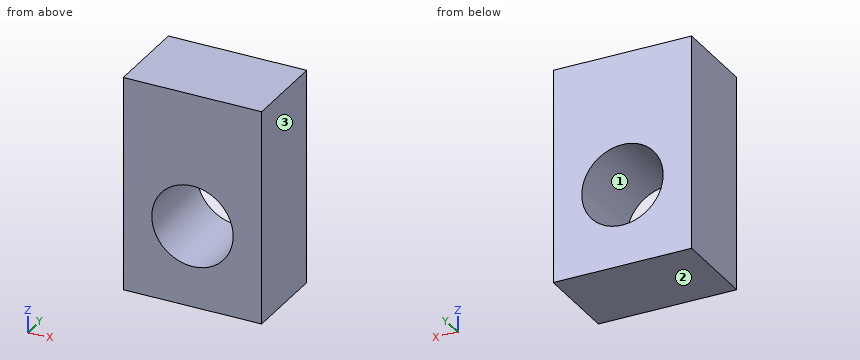
Autodesk Fusion 360 part; units mm, degrees
sketch "Sketch1" plane through (0, 0, 0) normal (0, 1, 0) x (1, 0, 0)
  line L0 (0, 0) -> (5.1, 0)
  line L1 (5.1, 0) -> (5.1, -7.9)
  line L2 (5.1, -7.9) -> (0, -7.9)
  line L3 (0, -7.9) -> (0, 0)
  point P0 (2.55, -3)
  dimension "d1" = 5.1
  dimension "d2" = 7.9
  dimension "d5" = 2.55
  dimension "d6" = 3
extrude "Extrude1" add sketch "Sketch1" along normal blind 3.2
hole "Hole1" at (2.55, 0, 3) direction (0, 1, 0) diameter 3 depth 8 tip angle 118
equation "d5 = ( 5.1 / 2 ) * 1 mm"
The model under review builds one solid part; all positions refer to its coordinate system, in mm. Face numbers are marked on the shaded views. Give positions to 0.01 mm unless a question says otherwise; leave off trailing zeros. Loops run counter-clockwise (first coordinate to the right, second up) from the corner with the lowest first, then second, coordinate; pieces in that order, holes last. Notation, with made-up numbers: (50.25, -18.5) -> (72.25, -18.5) arc R14 ccw to (72.25, -8.5) -> close; hole circle Ø2 at (37.5, 22.25). An arc over 180 degrees is marked (long way). Put each result on its own line as item: value. Start each with the question number.
1. We need section C-C on y = 0.35. State the section outline as (x, z) points.
2. Mouldability with a two-part tool opening along X and no side actions: class the marked faces 1, 2 and 3 as released by +X, released by -X, zero draft, split by the parting line, or undercut.
3. We need section A-A on z = 3. State the section outline as (x, y) points.
4. Clearance check with a flat-ended pin moving along its axis: P1, Ø2.5, axis at x = 2.55, z = 3, coming from the +Y side. State where the tip first meets the part, or that it passes through.
5. We need section B-B on x = 2.55. State the section outline as (y, z) points.
6. Wall thickness on probe 1 along X at (y, z) = (1.8, 3); probe 2 along Z at (x, y) = (2.55, 1.9); probe 3 along Z at (x, y) = (3, 0.75): over which ranges is each line inside the solid? List them lowest first.
Determined:
1. outline: (0, 0) -> (5.1, 0) -> (5.1, 7.9) -> (0, 7.9) -> close; hole circle Ø3 at (2.55, 3)
2. face 1: undercut
2. face 2: zero draft
2. face 3: released by +X
3. outline: (0, 0) -> (1.05, 0) -> (1.05, 3.2) -> (0, 3.2) -> close; (4.05, 0) -> (5.1, 0) -> (5.1, 3.2) -> (4.05, 3.2) -> close
4. P1: through
5. outline: (0, 0) -> (3.2, 0) -> (3.2, 1.5) -> (0, 1.5) -> close; (0, 4.5) -> (3.2, 4.5) -> (3.2, 7.9) -> (0, 7.9) -> close
6. probe 1: 0 to 1.05, 4.05 to 5.1
6. probe 2: 0 to 1.5, 4.5 to 7.9
6. probe 3: 0 to 1.57, 4.43 to 7.9
